For this review, take the finished solid that the model builds, in its own axes (mm). A direction names the side the tool comes from. Round coordinates to 2 decimals unless told otherwise and drop trailing zeros. Write each loop counter-clockwise with the first axis right and the second up, starting at its lowest first coordinate (ties: lowest second). Pieces come first, ordered by that corner, then holes. Notation, with made-up numbers: (42.25, 15) -> (61.25, 15) arc R26 ccw to (61.25, 51) -> close; hole circle Ø4 at (-19.75, 69). An arc over 180 degrees is marked (long way). Answer as CSV lines item,"result". Start each with the question number.
Item 1: Take a section at D-D on z = -9.5. Give the boundary of the cut face in (x, y).
Item 2: Take a section at A-A on y = 0. Give the boundary of the cut face in (x, z), then the cut area to 3 significant figures.
Item 3: Wall thickness on probe 1 along Y at (x, z) = (0, -10.85); probe 2 along Z at (x, y) = (1, 0.75); probe 3 along Z at (x, y) = (1.5, 2.5): over which ranges is each line inside the solid? List them lowest first. Write a range as from..to.
Item 4: Mouldability with a two-part tool opening along Y and no side actions: class faces 4 (the cylindrical face through (3.233, -1.341, 1.06)), 5 (the flat face through (1, -1, -11.35)), 6 (the cylindrical face through (-0.75, -0.03, -10.36)) as +Y half, -Y half, draft (parallel to the pull), parting line (faces both ways), or undercut.
Item 5: Machinability: for faces 1 (the flat face through (-1, 3, 2.15)), 2 (the flat face through (1, -1, -9.35)), 3 (the flat face through (-3, -1, 0)), which of the approach directions +Z, -Z, +X, -X, +Y, -Y give a long, thin tool a straight path to every point of the face, cutting with its end or side? Answer none if there is none.
Item 6: For pin 1 Ø1.4 at (x, y) = (0, 0) entering from +Z; pin 2 Ø1.5 at (y, z) = (2, -3) entering from +X; pin 3 Ø1 at (x, z) = (-2, -1) entering from +Y; pin 4 Ø1.5 at (y, z) = (1, -7.5) entering from -X, all flat-tipped, find the tip position at first contact; note any pin that passes through.
Item 7: Take a section at C-C on x = 1. Give the boundary of the cut face in (y, z), then the cut area to 3 significant figures.
```python
from build123d import *

# Parameters (mm, degrees)
F0_R     = 3.5
F1_DEPTH = 2.15
F2_R     = 2.75
F3_DEPTH = 11.35
F4_R     = 2.65
F5_DEPTH = 11.5
F6_R     = 0.75
F7_DEPTH = 13.501


with BuildPart() as f1:
    # F0 (on Top) → F1 (new body)
    with BuildSketch(Plane.XY):
        Circle(F0_R)
    extrude(amount=F1_DEPTH)

    # F2 (on Top) → F3 (join)
    with BuildSketch(Plane.XY):
        Circle(F2_R)
    extrude(amount=-F3_DEPTH)

    # F4 (on face) → F5 (cut)
    with BuildSketch(Plane.XY.offset(2.15)):
        Circle(F4_R)
    extrude(amount=-F5_DEPTH, mode=Mode.SUBTRACT)

    # F6 (on face) → F7 (cut, through all)
    with BuildSketch(Plane(origin=(0, 0, -11.35), x_dir=(1, 0, 0), z_dir=(0, 0, -1))):
        Circle(F6_R)
    extrude(amount=-F7_DEPTH, mode=Mode.SUBTRACT)


solid = f1.part
```
Output values:
1,outline,"circle Ø5.5 at (0, 0); hole circle Ø1.5 at (0, 0)"
2,outline,"(-3.5, 0) -> (-2.75, 0) -> (-2.75, -11.35) -> (-0.75, -11.35) -> (-0.75, -9.35) -> (-2.65, -9.35) -> (-2.65, 2.15) -> (-3.5, 2.15) -> close; (0.75, -11.35) -> (2.75, -11.35) -> (2.75, 0) -> (3.5, 0) -> (3.5, 2.15) -> (2.65, 2.15) -> (2.65, -9.35) -> (0.75, -9.35) -> close"
2,area,"13.5 mm^2"
3,probe 1,"y = -2.75..-0.75, 0.75..2.75"
3,probe 2,"z = -11.35..-9.35"
3,probe 3,"z = 0..2.15"
4,face 4,"parting line"
4,face 5,"draft"
4,face 6,"undercut"
5,face 1,"+Z, +X, -X, +Y, -Y"
5,face 2,"+Z"
5,face 3,"-Z"
6,pin 1,"passes through"
6,pin 2,"stops at x = 2.45"
6,pin 3,"stops at y = 2.3"
6,pin 4,"stops at x = -2.74"
7,outline,"(-3.35, 0) -> (-2.56, 0) -> (-2.56, -11.35) -> (2.56, -11.35) -> (2.56, 0) -> (3.35, 0) -> (3.35, 2.15) -> (2.45, 2.15) -> (2.45, -9.35) -> (-2.45, -9.35) -> (-2.45, 2.15) -> (-3.35, 2.15) -> close"
7,area,"16.1 mm^2"
